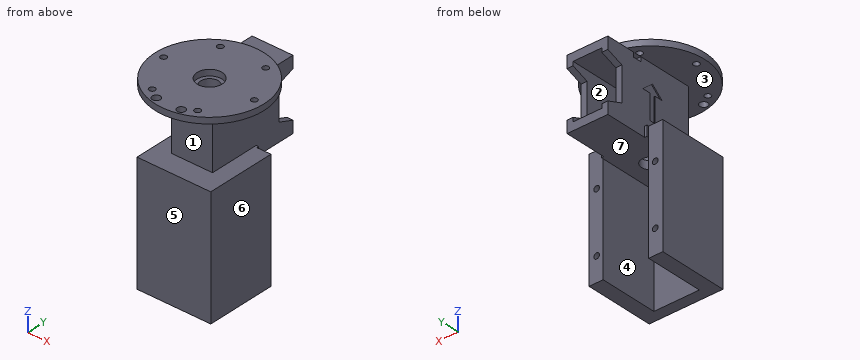
```python
from build123d import *

# Parameters (mm, degrees)
EXTRUDE_1_DEPTH     = 13.5
SKETCH_1_3_W        = 20.26
SKETCH_1_3_H        = 46
SKETCH_1_3_R        = 4.4
EXTRUDE_2_DEPTH     = 4
CUT_EXTRUDE_1_DEPTH = 40
CUT_EXTRUDE_2_DEPTH = 0.5
SKETCH_4_R          = 27
SKETCH_4_R_2        = 6.2
SKETCH_4_R_3        = 2
SKETCH_4_R_4        = 1.5
EXTRUDE_3_DEPTH     = 3
SKETCH_8_W          = 2.265156823
SKETCH_8_H          = 4.257571482
CUT_EXTRUDE_4_DEPTH = 30
EXTRUDE_11_DEPTH    = 5
EXTRUDE_12_DEPTH    = 5
EXTRUDE_13_DEPTH    = 54
SKETCH_13_R         = 1.4
CUT_EXTRUDE_5_DEPTH = 5
SKETCH_14_R         = 1.4
CUT_EXTRUDE_6_DEPTH = 5


with BuildPart() as part:
    # Sketch 1 → Extrude 1 (new body)
    with BuildSketch(Plane.XY):
        Polygon((-7.13, -7), (-4.13, -7), (-7.13, -4), (-7.13, 36), (-10.13, 36), (-10.13, -10), (-7.13, -10), align=None)
        Polygon((-7.13, -7), (-7.13, -10), (7.13, -10), (7.13, -7), (0, -7), align=None)
        Polygon((7.13, -4), (4.13, -7), (7.13, -7), (7.13, -10), (10.13, -10), (10.13, 36), (7.13, 36), align=None)
    extrude_1 = extrude(amount=EXTRUDE_1_DEPTH)

    # Sketch 1_3 → Extrude 2 (add)
    with BuildSketch(Plane.XY):
        with Locations((0, 13)):
            Rectangle(SKETCH_1_3_W, SKETCH_1_3_H)
        Circle(SKETCH_1_3_R, mode=Mode.SUBTRACT)
    extrude_2 = extrude(amount=-EXTRUDE_2_DEPTH)

    # Mirror 1: Extrude 1, Extrude 2 across plane
    add(extrude_1.mirror(Plane.XY.offset(13.5)))
    add(extrude_2.mirror(Plane.XY.offset(13.5)))

    # Sketch 2 → Cut-Extrude 1 (cut)
    with BuildSketch(Plane.ZY.offset(10.13)):
        Polygon((2, 36), (5, 28), (22, 28), (25, 36), align=None)
    extrude(amount=-CUT_EXTRUDE_1_DEPTH, mode=Mode.SUBTRACT)

    # Sketch 3 → Cut-Extrude 2 (cut)
    with BuildSketch(Plane.ZY.offset(10.13)):
        Polygon((5, 12), (17.297318311, 12), (17.297318311, 16), (22, 10.5), (17.297318311, 5), (17.297318311, 9), (5, 9), align=None)
    extrude(amount=-CUT_EXTRUDE_2_DEPTH, mode=Mode.SUBTRACT)

    # Sketch 4 → Extrude 3 (add)
    with BuildSketch(Plane.XY.offset(31)):
        Circle(SKETCH_4_R)
        Circle(SKETCH_4_R_2, mode=Mode.SUBTRACT)
        with Locations((6.088327702, -23.309373565)):
            Circle(SKETCH_4_R_3, mode=Mode.SUBTRACT)
        with Locations((22.434887901, -0.282877885)):
            Circle(SKETCH_4_R_4, mode=Mode.SUBTRACT)
        with Locations((11.179706516, 19.211668123)):
            Circle(SKETCH_4_R_4, mode=Mode.SUBTRACT)
        with Locations((-11.330656255, 19.211668123)):
            Circle(SKETCH_4_R_4, mode=Mode.SUBTRACT)
        with Locations((-22.58583764, -0.282877885)):
            Circle(SKETCH_4_R_4, mode=Mode.SUBTRACT)
        with Locations((-11.330656255, -19.777423893)):
            Circle(SKETCH_4_R_4, mode=Mode.SUBTRACT)
        with Locations((11.179706516, -19.777423893)):
            Circle(SKETCH_4_R_4, mode=Mode.SUBTRACT)
        with Locations((-6.239277441, -23.309373565)):
            Circle(SKETCH_4_R_3, mode=Mode.SUBTRACT)
    extrude(amount=EXTRUDE_3_DEPTH)

    # Sketch 8 → Cut-Extrude 4 (cut)
    with BuildSketch(Plane(origin=(-10.13, 0, 0.991647231), x_dir=(0, 0, 1), z_dir=(-1, 0, 0))):
        with Locations((28.867421589, 19.251576228)):
            Rectangle(SKETCH_8_W, SKETCH_8_H)
    extrude(amount=-CUT_EXTRUDE_4_DEPTH, mode=Mode.SUBTRACT)

    # Sketch 11 → Extrude 11 (add)
    with BuildSketch(Plane(origin=(0, 0, -4), x_dir=(-1, 0, 0), z_dir=(0, 0, -1))):
        Polygon((11.3, 0), (10.13, 0), (10.13, -10), (-10.13, -10), (-10.13, 15), (-11.3, 15), (-11.3, 14), (-11.3, -15), (11.3, -15), align=None)
        Polygon((10.13, 15), (10.13, 0), (11.3, 0), (11.3, 14), (11.3, 15), align=None)
    extrude(amount=-EXTRUDE_11_DEPTH)

    # Sketch 11_3 → Extrude 12 (add)
    with BuildSketch(Plane(origin=(0, 0, -4), x_dir=(-1, 0, 0), z_dir=(0, 0, -1))):
        Polygon((11.3, 14), (11.3, 0), (11.3, -15), (-11.3, -15), (-11.3, 14), (-18.3, 14), (-18.3, -17.416972989), (-18.3, -20.416972989), (18.3, -20.416972989), (18.3, 14), align=None)
    extrude(amount=-EXTRUDE_12_DEPTH)

    # Sketch 11_4 → Extrude 13 (add)
    with BuildSketch(Plane(origin=(0, 0, -4), x_dir=(-1, 0, 0), z_dir=(0, 0, -1))):
        Polygon((11.3, 14), (11.3, 0), (11.3, -15), (-11.3, -15), (-11.3, 14), (-18.3, 14), (-18.3, -17.416972989), (-18.3, -20.416972989), (18.3, -20.416972989), (18.3, 14), align=None)
    extrude(amount=EXTRUDE_13_DEPTH)

    # Sketch 13 → Cut-Extrude 5 (cut)
    with BuildSketch(Plane(origin=(0, 14, 0), x_dir=(1, 0, 0), z_dir=(0, 1, 0))):
        with Locations((-14.55, 16)):
            Circle(SKETCH_13_R)
        with Locations((-14.55, 46)):
            Circle(SKETCH_13_R)
    extrude(amount=-CUT_EXTRUDE_5_DEPTH, mode=Mode.SUBTRACT)

    # Sketch 14 → Cut-Extrude 6 (cut)
    with BuildSketch(Plane(origin=(0, 14, 0), x_dir=(1, 0, 0), z_dir=(0, 1, 0))):
        with Locations((14.55, 16)):
            Circle(SKETCH_14_R)
        with Locations((14.55, 46)):
            Circle(SKETCH_14_R)
    extrude(amount=-CUT_EXTRUDE_6_DEPTH, mode=Mode.SUBTRACT)


solid = part.part
```
Can you work these out from the model? Positions are in its coordinate system, mm. Face numbers are marked on the shaded views. A direction names the side the tool comes from. Round coordinates to 2 decimals unless told otherwise and drop trailing zeros. Loops run counter-clockwise (first coordinate to the right, second up) from the corner with the lowest first, then second, coordinate; pieces in that order, holes last. Notation, with made-up numbers: M -35.75,-6 L -29.75,-6 A18 ccw -29.75,5 Z; hole C 87,-35.5 d10. An arc over 180 degrees is marked long. Answer as a JSON object with one key per item and string values. Group by question number.
Q1. On a 3-axis mill with a long thin cutter (end or side, diameter ignored), from which of +Z, -Z, +X, -X, +Y, -Y can I reach the whole of each face in a straight line? I mean the marked faces 1, 2, 3 and 4. Say none if no direction works.
Q2. Will these pins go through, and if not, where does the flat tip stop? pin 1 (12 mm diameter, centred on x = 19.5, z = -28.5, fed in from +Y); pin 2 (6 mm diameter, centred on y = 4, z = 12, fed in from -X); pin 3 (23 mm diameter, centred on y = -4, z = -25.5, fed in from -X).
Q3. Imagine slicing it at A-A, the plane z = -3. Please give me the cut outline in (x, y), then the cut area to 3 significant figures.
Q4. Imagine slicing it at C-C, the plane x = 0.5. Count the separate pieces of the cut face and the enclosed holes in it, then the cut area to 3 significant figures.
Q5. Imagine slicing it at D-D, the plane z = -16. Please give me the cut outline in (x, y).
Q6. Please list where these lines run through material, in increasing order: L1, parallel to X at y = 12, z = -16; L2, parallel to Z at x = -7, y = 18; L3, parallel to Z at x = -12, y = 7.5.
Q7. We'd pull the mould along X, two halves only. Please class the marked faces 5, 6 and 7: +X half, -X half, draft (parallel to the pull), parting line (faces both ways), or undercut.
Q8. Imagine slicing it at B-B, the plane y = 13. Please give me the cut outline in (x, z).
Findings:
{
 "1": {"face 1": "+X, -X, -Y", "face 2": "+Y", "face 3": "-Y", "face 4": "-Z, +Y"},
 "2": {"pin 1": "stops at y = 14", "pin 2": "stops at x = -10.13", "pin 3": "stops at x = -18.3"},
 "3": {"outline": "M -18.3,-20.42 L 18.3,-20.42 L 18.3,14 L 11.3,14 L 11.3,15 L 10.13,15 L 10.13,36 L -10.13,36 L -10.13,15 L -11.3,15 L -11.3,14 L -18.3,14 Z; hole C 0,0 d8.8", "area": "1,650 mm2"},
 "4": {"separate pieces": "3", "enclosed holes": "1", "area": "839 mm2"},
 "5": {"outline": "M -18.3,-20.42 L 18.3,-20.42 L 18.3,14 L 15.95,14 L 15.95,9 L 13.15,9 L 13.15,14 L 11.3,14 L 11.3,-15 L -11.3,-15 L -11.3,14 L -13.15,14 L -13.15,9 L -15.95,9 L -15.95,14 L -18.3,14 Z"},
 "6": {"L1": "x = -18.3 to -15.95, -13.15 to -11.3, 11.3 to 13.15, 15.95 to 18.3", "L2": "z = -4 to 0, 27 to 28.73, 30.99 to 34", "L3": "z = -58 to 1, 31 to 34"},
 "7": {"face 5": "draft", "face 6": "+X half", "face 7": "undercut"},
 "8": {"outline": "M -23.66,31 L -10.13,31 L -10.13,19.86 L -9.63,19.86 L -9.63,17.3 L -10.13,17.3 L -10.13,1 L -18.3,1 L -18.3,-58 L -11.3,-58 L -11.3,-4 L 11.3,-4 L 11.3,-58 L 18.3,-58 L 18.3,1 L 10.13,1 L 10.13,31 L 23.66,31 L 23.66,34 L -23.66,34 Z; hole C -14.55,-46 d2.8; hole C -14.55,-16 d2.8; hole M -7.13,0 L 7.13,0 L 7.13,27 L -7.13,27 Z; hole C 14.55,-46 d2.8; hole C 14.55,-16 d2.8"}
}
